Study the drawing (mm; zero at the part's minimum x, y, z) and answer. Coordinates: 2 decimals unless noted, no trailing zeros. Order: outer loops, then holes, each group sorted by start corner. A loop starts at its lowest first (then second) coordinate and runs counter-clockwise, first axis right, second up. Notation, with made-up numbers: (73, -5) -> (96, -5) arc R16 cw to (96, 0) -> close; hole circle Ø2 at (-35.5, -25.75). An arc over 180 degrees is marked (long way). Answer as CSV lines item,"result". Start each with the question number.
Item 1: Straight lines are drawn through the part: L1, parallel to X at y = 0.7, z = 42.95; L2, parallel to Z at x = 180.7, y = 2; L3, parallel to Z at x = 9, y = 1.7. For each, find the intervals that lie inside material, in ascending order.
Item 2: Section A-A (x = 180.7) is taken. Write down the section's boundary in (y, z) (3 decimals), then the cut area to 3 significant figures.
Item 3: Section B-B (z = 211.05) is taken. Write down the section's boundary in (x, y) (3 decimals).
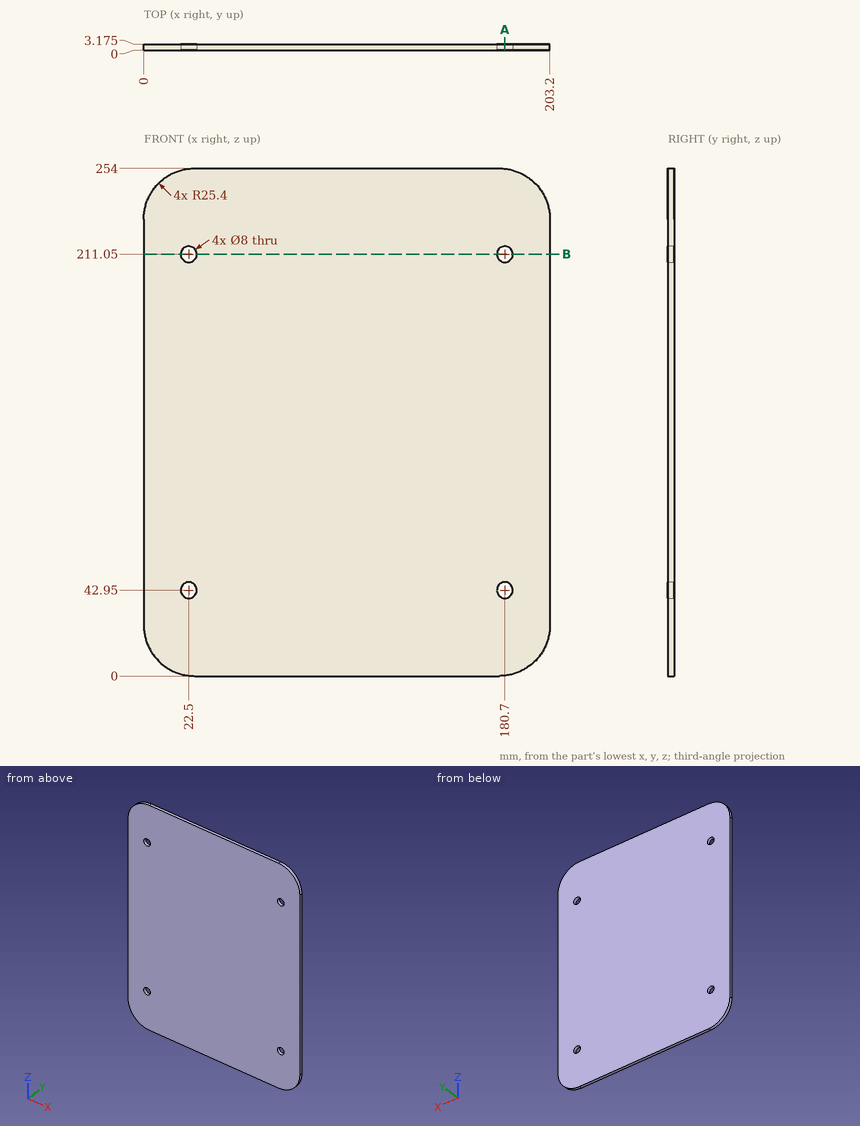
Checked values:
1,L1,"x = 0 to 18.5, 26.5 to 176.7, 184.7 to 203.2"
1,L2,"z = 0.17 to 38.95, 46.95 to 207.05, 215.05 to 253.83"
1,L3,"z = 6 to 248"
2,outline,"(0, 0.166) -> (3.175, 0.166) -> (3.175, 38.95) -> (0, 38.95) -> close; (0, 46.95) -> (3.175, 46.95) -> (3.175, 207.05) -> (0, 207.05) -> close; (0, 215.05) -> (3.175, 215.05) -> (3.175, 253.834) -> (0, 253.834) -> close"
2,area,"755 mm^2"
3,outline,"(0, 0) -> (18.5, 0) -> (18.5, 3.175) -> (0, 3.175) -> close; (26.5, 0) -> (176.7, 0) -> (176.7, 3.175) -> (26.5, 3.175) -> close; (184.7, 0) -> (203.2, 0) -> (203.2, 3.175) -> (184.7, 3.175) -> close"
